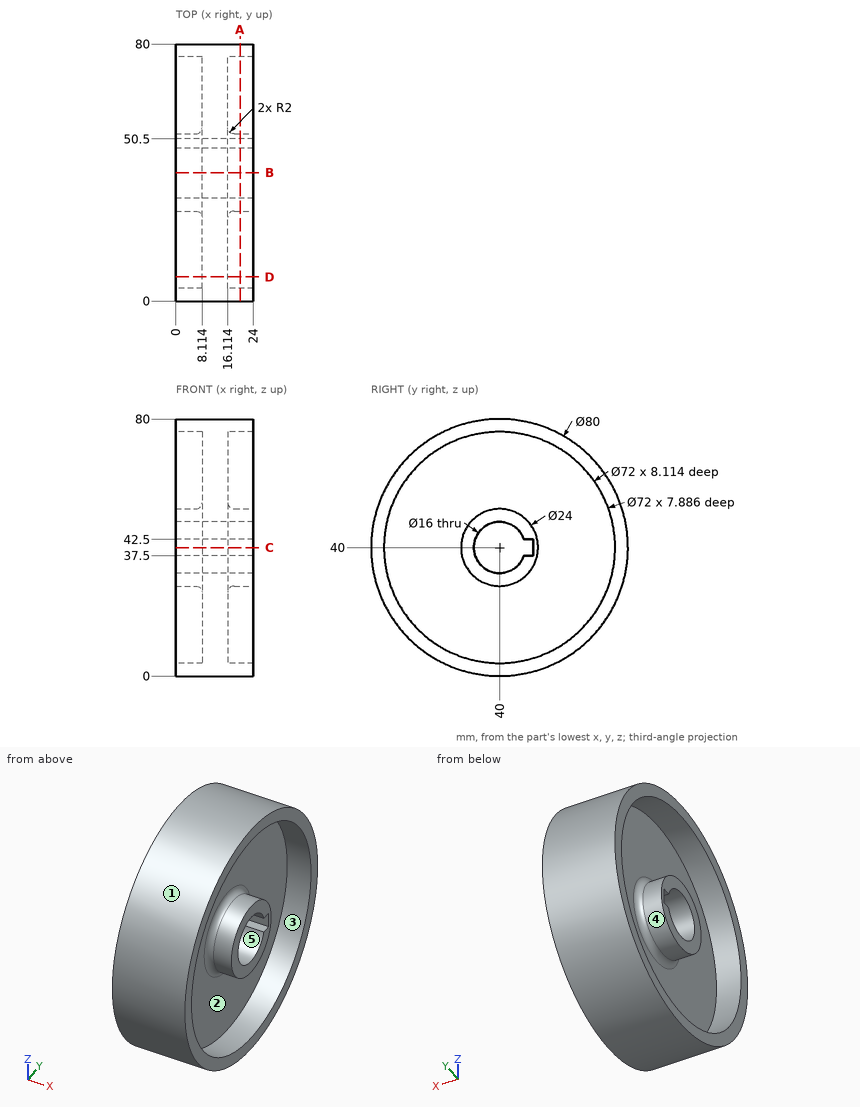
Geometry check sheet. Reference: drawing and pictorial views, mm from the part's lowest x, y, z. A direction names the side the tool comes from. Round coordinates to 2 decimals unless told otherwise and drop trailing zeros. Loops run counter-clockwise (first coordinate to the right, second up) from the corner with the lowest first, then second, coordinate; pieces in that order, holes last. Notation, with made-up numbers: (45, -22) - (104, -22) arc R25 cw to (104, 0) - close; hole circle Ø5 at (4.5, -19.75). An arc over 180 degrees is marked (long way). Write item = value, one per line. Start each with the question number.
Q1. Access from +Z, -Z, +X, -X, +Y, -Y to the whole of each face (thin tool, end or side, straight path). Record for the marked faces 3, 4 and 5.
Q2. Depth check by flat-ended pin: P1, Ø12, axis at y = 65, z = 32.5, coming from the -X side; P2, Ø3, axis at x = 15, y = 22.5, coming from the +Z side; P3, Ø10, axis at y = 50, z = 55.5, coming from the -X side; P4, Ø2, axis at x = 13, y = 40.5, coming from the +Z side. Enter the tip coordinate at first touch or a pass-through.
Q3. Release check for a two-part mould opening along Z. For the marked faces 1 and 2 record: pulls with the +Z half, pulls with the -Z half, needs draft (parallel to the pull), parting line crosses it, or undercut.
Q4. Thickness scan on L1, parallel to Y at x = 19.5, z = 40; L2, parallel to Y at x = 6.75, z = 40; L3, parallel to Z at x = 21, y = 24. Record the ranges inside material, lowest first.
Q5. Section check A-A (x = 20). Record the boundary of the cut face in (y, z).
Q6. Section check B-B (y = 40). Record the boundary of the cut face in (x, z).
Q7. Section check C-C (z = 40). Record the boundary of the cut face in (x, y).
Q8. Section check D-D (y = 7.5). Record the boundary of the cut face in (x, z), plus the area to 3 significant figures.
Derived:
q1.face_3 = +X
q1.face_4 = -X
q1.face_5 = +X, -X
q2.P1 = 8.11
q2.P2 = 76.66
q2.P3 = 8.04
q2.P4 = 80
q3.face_1 = parting line crosses it
q3.face_2 = undercut
q4.L1 = 0 to 4, 28 to 32, 50.5 to 52, 76 to 80
q4.L2 = 0 to 4, 27.9 to 32, 50.5 to 52.1, 76 to 80
q4.L3 = 3.34 to 7.75, 72.25 to 76.66
q5.outline = circle Ø80 at (40, 40); circle Ø24 at (40, 40); hole circle Ø72 at (40, 40); hole (47.6, 37.5) - (50.5, 37.5) - (50.5, 42.5) - (47.6, 42.5) arc R8 ccw (long way) to start
q6.outline = (0, 0) - (24, 0) - (24, 4) - (16.11, 4) - (16.11, 26) arc R2 cw to (18.11, 28) - (24, 28) - (24, 32) - (0, 32) - (0, 28) - (6.11, 28) arc R2 cw to (8.11, 26) - (8.11, 4) - (0, 4) - close; (0, 48) - (24, 48) - (24, 52) - (18.11, 52) arc R2 cw to (16.11, 54) - (16.11, 76) - (24, 76) - (24, 80) - (0, 80) - (0, 76) - (8.11, 76) - (8.11, 54) arc R2 cw to (6.11, 52) - (0, 52) - close
q7.outline = (0, 0) - (24, 0) - (24, 4) - (16.11, 4) - (16.11, 26) arc R2 cw to (18.11, 28) - (24, 28) - (24, 32) - (0, 32) - (0, 28) - (6.11, 28) arc R2 cw to (8.11, 26) - (8.11, 4) - (0, 4) - close; (0, 50.5) - (24, 50.5) - (24, 52) - (18.11, 52) arc R2 cw to (16.11, 54) - (16.11, 76) - (24, 76) - (24, 80) - (0, 80) - (0, 76) - (8.11, 76) - (8.11, 54) arc R2 cw to (6.11, 52) - (0, 52) - close
q8.outline = (0, 16.68) - (24, 16.68) - (24, 24.52) - (16.11, 24.52) - (16.11, 55.48) - (24, 55.48) - (24, 63.32) - (0, 63.32) - (0, 55.48) - (8.11, 55.48) - (8.11, 24.52) - (0, 24.52) - close
q8.area = 624 mm^2
